Part model, mm, in its own coordinate system. Face numbers are marked on the shaded views. Round coordinates to 2 decimals unless told otherwise and drop trailing zeros. Loops run counter-clockwise (first coordinate to the right, second up) from the corner with the lowest first, then second, coordinate; pieces in that order, holes last. Notation, with made-up numbers: M 38,-38.5 L 55,-38.5 A18 cw 55,-5.5 Z; hole C 50.25,37.25 d1. An arc over 180 degrees is marked long. Put each result on its own line as item: value. Start each with the question number.
1) Slice it at C-C on z = 2.05. State how many separate pieces and enclosed holes the cut face has, then the cut area to 3 significant figures.
2) Pull direction Z, two halves, no side cores. Call the marked faces 1 and 2: +Z half, -Z half, draft (parallel to the pull), parting line (faces both ways), or undercut.
3) Slice it at B-B on x = -88.5. Give the cut face in (y, z), then the cut area to 3 significant figures.
4) Probe line 1 along X through (y, z) = (2.5, 2.65); line 2 along X through (y, z) = (7, 2.65); line 3 along Y through (x, z) = (-109.5, 1.85). List the from-to ranges inside material, lowest first.
5) Slice it at A-A on y = 21.5. Give the cut face in (x, z), then the cut area to 3 significant figures.
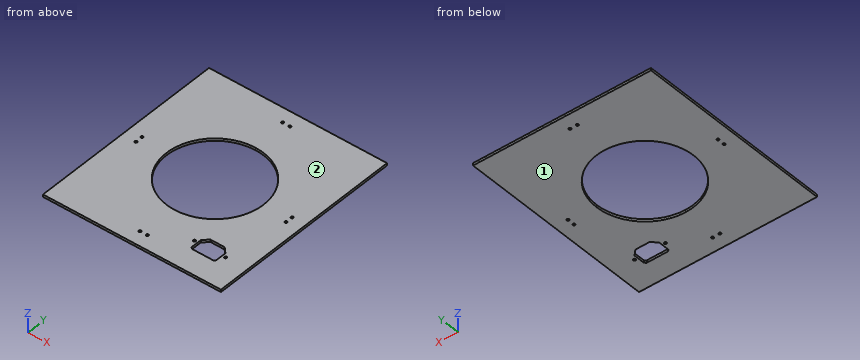
```python
from build123d import *

# Parameters (mm, degrees)
SKETCH1_W           = 210
SKETCH1_H           = 245
BOSS_EXTRUDE1_DEPTH = 3
CUT_EXTRUDE1_DEPTH  = 3
CUT_EXTRUDE2_DEPTH  = 3
CUT_EXTRUDE3_DEPTH  = 246.456036562
SKETCH5_W           = 3
SKETCH5_H           = 245
BOSS_EXTRUDE2_DEPTH = 5
SKETCH6_W           = 3
SKETCH6_H           = 245
BOSS_EXTRUDE3_DEPTH = 5
SKETCH7_R           = 1.5
CUT_EXTRUDE4_DEPTH  = 10


with BuildPart() as part:
    # Sketch1 → Boss-Extrude1 (new body)
    with BuildSketch(Plane.XY):
        with Locations((-105, 4.541984733)):
            Rectangle(SKETCH1_W, SKETCH1_H)
    extrude(amount=BOSS_EXTRUDE1_DEPTH)

    # Sketch2 → Cut-Extrude1 (cut)
    with BuildSketch(Plane.XY.offset(3)):
        with BuildLine():
            ThreePointArc((-45, 4.541984733), (-62.573593129, 46.968391604), (-105, 64.541984733))
            Line((-105, 64.541984733), (-105, -55.458015267))
            ThreePointArc((-105, -55.458015267), (-62.573593129, -37.884422138), (-45, 4.541984733))
        make_face()
        with BuildLine():
            Line((-105, -55.458015267), (-105, 64.541984733))
            ThreePointArc((-105, 64.541984733), (-165, 4.541984733), (-105, -55.458015267))
        make_face()
    extrude(amount=-CUT_EXTRUDE1_DEPTH, mode=Mode.SUBTRACT)

    # Sketch3 → Cut-Extrude2 (cut)
    with BuildSketch(Plane.XY.offset(3)):
        Polygon((-41.653041136, -88.602014661), (-41.653041136, -68.081199381), (-50.153041136, -68.081199381), (-56.163448776, -74.091607021), (-56.163448776, -87.091607021), (-54.653041136, -88.602014661), align=None)
        Polygon((-41.653041136, -68.081199381), (-41.653041136, -67.381199381), (-50.442990629, -67.381199381), (-56.863448776, -73.801657527), (-56.863448776, -87.381556515), (-54.942990629, -89.302014661), (-41.653041136, -89.302014661), (-41.653041136, -88.602014661), (-54.653041136, -88.602014661), (-56.163448776, -87.091607021), (-56.163448776, -74.091607021), (-50.153041136, -68.081199381), align=None)
        Polygon((-33.153041136, -68.081199381), (-41.653041136, -68.081199381), (-41.653041136, -88.602014661), (-28.653041136, -88.602014661), (-27.142633496, -87.091607021), (-27.142633496, -74.091607021), align=None)
        Polygon((-32.863091642, -67.381199381), (-41.653041136, -67.381199381), (-41.653041136, -68.081199381), (-33.153041136, -68.081199381), (-27.142633496, -74.091607021), (-27.142633496, -87.091607021), (-28.653041136, -88.602014661), (-41.653041136, -88.602014661), (-41.653041136, -89.302014661), (-28.363091642, -89.302014661), (-26.442633496, -87.381556515), (-26.442633496, -73.801657527), align=None)
    extrude(amount=-CUT_EXTRUDE2_DEPTH, mode=Mode.SUBTRACT)

    # Sketch4 → Cut-Extrude3 (cut, through all)
    with BuildSketch(Plane.XY.offset(3)):
        with BuildLine():
            ThreePointArc((-60.863448776, -76.841607021), (-62.363448776, -78.341607021), (-60.863448776, -79.841607021))
            Line((-60.863448776, -79.841607021), (-60.863448776, -76.841607021))
        make_face()
        with BuildLine():
            Line((-60.863448776, -76.841607021), (-60.863448776, -79.841607021))
            ThreePointArc((-60.863448776, -79.841607021), (-59.802788604, -79.402267193), (-59.363448776, -78.341607021))
            ThreePointArc((-59.363448776, -78.341607021), (-59.802788604, -77.280946849), (-60.863448776, -76.841607021))
        make_face()
        with BuildLine():
            ThreePointArc((-22.442633496, -76.841607021), (-23.942633496, -78.341607021), (-22.442633496, -79.841607021))
            Line((-22.442633496, -79.841607021), (-22.442633496, -76.841607021))
        make_face()
        with BuildLine():
            Line((-22.442633496, -76.841607021), (-22.442633496, -79.841607021))
            ThreePointArc((-22.442633496, -79.841607021), (-21.381973324, -79.402267193), (-20.942633496, -78.341607021))
            ThreePointArc((-20.942633496, -78.341607021), (-21.381973324, -77.280946849), (-22.442633496, -76.841607021))
        make_face()
    extrude(amount=-CUT_EXTRUDE3_DEPTH, mode=Mode.SUBTRACT)

    # Sketch5 → Boss-Extrude2 (add)
    with BuildSketch(Plane(origin=(0, 0, 0), x_dir=(0, 0, -1), z_dir=(1, 0, 0))):
        with Locations((-1.5, 4.541984733)):
            Rectangle(SKETCH5_W, SKETCH5_H)
    extrude(amount=BOSS_EXTRUDE2_DEPTH)

    # Sketch6 → Boss-Extrude3 (add)
    with BuildSketch(Plane.ZY.offset(210)):
        with Locations((1.5, 4.541984733)):
            Rectangle(SKETCH6_W, SKETCH6_H)
    extrude(amount=BOSS_EXTRUDE3_DEPTH)

    # Sketch7 → Cut-Extrude4 (cut)
    with BuildSketch(Plane(origin=(0, 0, 0), x_dir=(-1, 0, 0), z_dir=(0, 0, -1))):
        with Locations((100.5, -100.70506409)):
            Circle(SKETCH7_R)
        with Locations((100.5, 109.789033556)):
            Circle(SKETCH7_R)
        with Locations((12.252951177, -1.473015267)):
            Circle(SKETCH7_R)
        with Locations((12.252951177, 7.526984733)):
            Circle(SKETCH7_R)
        with Locations((109.5, -100.70506409)):
            Circle(SKETCH7_R)
        with Locations((109.5, 109.789033556)):
            Circle(SKETCH7_R)
        with Locations((197.747048823, -1.473015267)):
            Circle(SKETCH7_R)
        with Locations((197.747048823, 7.526984733)):
            Circle(SKETCH7_R)
    extrude(amount=-CUT_EXTRUDE4_DEPTH, mode=Mode.SUBTRACT)


solid = part.part
```
Recorded:
1. separate pieces: 1
1. enclosed holes: 12
1. area: 41,900 mm2
2. face 1: -Z half
2. face 2: +Z half
3. outline: M -117.96,0 L -53.14,0 L -53.14,3 L -117.96,3 Z; M 62.23,0 L 127.04,0 L 127.04,3 L 62.23,3 Z
3. area: 389 mm2
4. line 1: x = -215 to -164.97, -45.03 to 5
4. line 2: x = -215 to -199.15, -196.34 to -164.95, -45.05 to -13.66, -10.85 to 5
4. line 3: y = -117.96 to -102.21, -99.21 to -55.29, 64.37 to 108.29, 111.29 to 127.04
5. outline: M -215,0 L -162.55,0 L -162.55,3 L -215,3 Z; M -47.45,0 L 5,0 L 5,3 L -47.45,3 Z
5. area: 315 mm2
